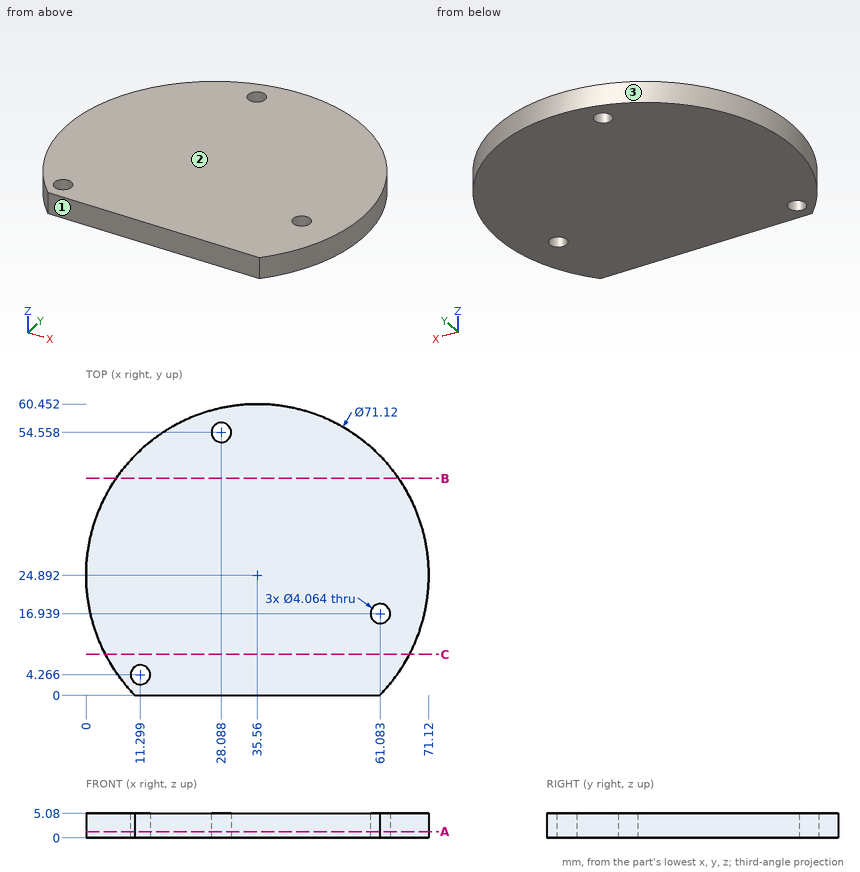
Design review of the part shown in the three views and the two pictorial views. Dimensions are in mm from the part's minimum x, y and z. Round coordinates to 2 decimals unless told otherwise and drop trailing zeros. Write each loop counter-clockwise with the first axis right and the second up, starting at its lowest first coordinate (ties: lowest second). Pieces come first, ordered by that corner, then holes.
Item 1: We need section A-A on z = 1.25. Write out the cut boundary in (x, y) (1 decimal), and give its area (3 significant figures).
Item 2: We need section B-B on y = 45. Write out the cut boundary in (x, z), and give its area (3 significant figures).
Item 3: For probe 1 along X at (y, z) = (53, 3.85) (1 decimal); probe 2 along Y at (x, z) = (13, 1.7) (1 decimal); probe 3 along X at (y, z) = (24, 3.25), list the stretches that pass through material, from the lowest coordinate up.
Item 4: The part is to be moulded in two halves that separate along Y. For the marked faces 1, 2 and 3, say which applies: +Y half, -Y half, draft (parallel to the pull), parting line (faces both ways), or undercut.
Item 5: Clearance check with flat-ended pins moving along their axes: pin 1 Ø2.5 at (x, y) = (11.3, 4.27) entering from +Z; pin 2 Ø2 at (x, z) = (47, 4) entering from +Y (1 decimal). State where each tip first meets the part, or that it passes through.
Item 6: We need section C-C on y = 8.5. Write out the cut boundary in (x, z).
Returned:
1. outline: (10.2, 0) - (61, 0) arc R35.6 ccw (long way) to start; hole circle Ø4.1 at (11.3, 4.3); hole circle Ø4.1 at (28.1, 54.6); hole circle Ø4.1 at (61.1, 16.9)
1. area: 3,560 mm2
2. outline: (6.23, 0) - (64.89, 0) - (64.89, 5.08) - (6.23, 5.08) - close
2. area: 298 mm2
3. probe 1: x = 13.8 to 26.8, 29.4 to 57.3
3. probe 2: y = 0 to 3.2, 5.4 to 52.4
3. probe 3: x = 0.01 to 71.11
4. face 1: -Y half
4. face 2: draft
4. face 3: parting line
5. pin 1: passes through
5. pin 2: stops at y = 58.9
6. outline: (4, 0) - (67.12, 0) - (67.12, 5.08) - (4, 5.08) - close
